Could you check a few things on this model? Use its own coordinates, in mm. A direction names the side the tool comes from. Coordinates: 2 decimals unless noted, no trailing zeros. Loops run counter-clockwise (first coordinate to the right, second up) from the corner with the lowest first, then second, coordinate; pieces in that order, holes last. Notation, with made-up numbers: (66, -37.75) - (77, -37.75) arc R24 ccw to (77, -1.75) - close; hole circle Ø10 at (33, 47). An arc over 180 degrees is marked (long way). Use CSV: the item, a comma, the result in double quotes.
from build123d import *

# Parameters (mm, degrees)
F1_DEPTH = 97.536
F2_R     = 28.207671


with BuildPart() as f1:
    # F0 (on Front) → F1 (new body)
    with BuildSketch(Plane.XZ):
        Polygon((-20.546786, 40.685356), (-45.039643, 40.685356), (-45.039643, 15.920358), (-53.748216, 15.920358), (-45.039643, -38.780358), (25.717502, -48.305355), (25.717502, -38.780358), (45.311786, -38.780358), (45.311786, 40.685356), (25.717502, 40.685356), (25.717502, 50.754644), (-20.546786, 50.754644), align=None)
    extrude(amount=F1_DEPTH)

    # F2
    f2_edges = [f1.edges().sort_by_distance(p)[0] for p in [
        (2.585358, -97.536, 50.754644),
    ]]
    fillet(f2_edges, radius=F2_R)


solid = f1.part
(1) Please list where these lines run through material, in increasing order: line 1 (X direction, y = -51, z = 33.5); line 2 (X direction, y = -53, z = 45); line 3 (Z direction, x = -14, y = -59).
Computed:
line 1,"x = -45.04 to 45.31"
line 2,"x = -20.55 to 25.72"
line 3,"z = -42.96 to 50.75"
(2) Suppose I cut it at C-C (x = -12.5). Write out the boundary of the cut face in (y, z), plus the area to 3 significant figures.
Computed:
outline,"(-97.54, -43.16) - (0, -43.16) - (0, 50.75) - (-69.33, 50.75) arc R28.21 ccw to (-97.54, 22.55) - close"
area,"8,990 mm²"
(3) Will these pins go through, and if not, where does the flat tip stop? pin 1 (3 mm diameter, centred on y = -24.5, z = 46.5, fed in from -X); pin 2 (12 mm diameter, centred on x = -30.5, y = -41.5, fed in from +Z); pin 3 (5 mm diameter, centred on x = -39, y = -11, fed in from -Z).
Computed:
pin 1,"stops at x = -20.55"
pin 2,"stops at z = 40.69"
pin 3,"stops at z = -39.93"
(4) Suppose I cut it at A-A (y = -33). Write out the boundary of the cut face in (x, z).
Computed:
outline,"(-53.75, 15.92) - (-45.04, -38.78) - (25.72, -48.31) - (25.72, -38.78) - (45.31, -38.78) - (45.31, 40.69) - (25.72, 40.69) - (25.72, 50.75) - (-20.55, 50.75) - (-20.55, 40.69) - (-45.04, 40.69) - (-45.04, 15.92) - close"
(5) Suppose I cut it at D-D (y = -81.5). Write out the boundary of the cut face in (x, z), plus the area to 3 significant figures.
Computed:
outline,"(-53.75, 15.92) - (-45.04, -38.78) - (25.72, -48.31) - (25.72, -38.78) - (45.31, -38.78) - (45.31, 40.69) - (25.72, 40.69) - (25.72, 47.99) - (-20.55, 47.99) - (-20.55, 40.69) - (-45.04, 40.69) - (-45.04, 15.92) - close"
area,"8,090 mm²"
(6) Suppose I cut it at B-B (z = 21). Write out the boundary of the cut face in (x, y), plus the area to 3 significant figures.
Computed:
outline,"(-45.04, -97.54) - (45.31, -97.54) - (45.31, 0) - (-45.04, 0) - close"
area,"8,810 mm²"
(7) Which directions (+Z, -Z, +X, -X, +Y, -Y) give clear straight access to the entire face, cutting with the end or side of a thin tool? Please do faces 1 (the face through (-33, -45, 40.685)), 2 (the face through (-10.156, -48.085, -43.476)), 3 (the face through (25.718, -48, -44)), 4 (the face through (45.312, -48, 0)), 5 (the face through (25.718, -45, 46)).
Computed:
face 1,"+Z, -X, +Y, -Y"
face 2,"-Z, -X, +Y, -Y"
face 3,"-Z, +X, +Y, -Y"
face 4,"+Z, -Z, +X, +Y, -Y"
face 5,"+Z, +X, +Y, -Y"
